```python
from build123d import *

# Parameters (mm, degrees)
SKETCH_1_W      = 20
SKETCH_1_H      = 20
EXTRUDE_1_DEPTH = 5
SKETCH_2_W      = 6
SKETCH_2_H      = 3
SKETCH_2_W_2    = 3
SKETCH_2_H_2    = 6
EXTRUDE_2_DEPTH = 15
SKETCH_3_W      = 6
SKETCH_3_H      = 3
EXTRUDE_3_DEPTH = 15
SKETCH_4_W      = 3
SKETCH_4_H      = 6
EXTRUDE_4_DEPTH = 15


with BuildPart() as part:
    # Эскиз1 → Бобышка-Вытянуть1 (new body)
    with BuildSketch(Plane.XY):
        with Locations((10, 10)):
            Rectangle(SKETCH_1_W, SKETCH_1_H)
    extrude(amount=EXTRUDE_1_DEPTH)

    # Эскиз2 → Бобышка-Вытянуть2 (add)
    with BuildSketch(Plane.XY.offset(5)):
        with Locations((10, 18.5)):
            Rectangle(SKETCH_2_W, SKETCH_2_H)
        with Locations((18.5, 10)):
            Rectangle(SKETCH_2_W_2, SKETCH_2_H_2)
    extrude(amount=EXTRUDE_2_DEPTH)

    # Эскиз3 → Бобышка-Вытянуть3 (add)
    with BuildSketch(Plane.XZ):
        with Locations((10, 1.5)):
            Rectangle(SKETCH_3_W, SKETCH_3_H)
    extrude(amount=EXTRUDE_3_DEPTH)

    # Эскиз4 → Бобышка-Вытянуть4 (add)
    with BuildSketch(Plane.ZY):
        with Locations((1.5, 10)):
            Rectangle(SKETCH_4_W, SKETCH_4_H)
    extrude(amount=EXTRUDE_4_DEPTH)


solid = part.part
```
The listing builds one solid part. Answer for the finished solid, in the listing's coordinates (mm). A direction names the side the tool comes from. Give positions to 0.01 mm unless a question says otherwise; leave off trailing zeros. Loops run counter-clockwise (first coordinate to the right, second up) from the corner with the lowest first, then second, coordinate; pieces in that order, holes last. Notation, with made-up numbers: (76, 26.25) - (108, 26.25) arc R22 ccw to (108, 37.25) - close; hole circle Ø7 at (71, 68.5). An arc over 180 degrees is marked (long way). Return JSON: item names as keys, results as strings. Group by question number.
1. Find section C-C (y = -6). Write down the section's boundary in (x, z).
2. Which of the six approach directions +Z, -Z, +X, -X, +Y, -Y give full straight-line access (tool end or side, diameter ignored) to faces 4 (the flat face through (18, 13, 12)), 5 (the flat face through (7, -7, 1)), 6 (the flat face through (7, 18, 12)), 7 (the flat face through (10, -7, 3))?
3. Given pin 1 Ø3 at (x, y) = (9.5, -5) entering from +Z; pin 2 Ø1.5 at (x, y) = (-3, 15.5) entering from -Z; pin 3 Ø0.9 at (x, z) = (18, 13.5) entering from +Y; pin 4 Ø1.5 at (x, z) = (18, 13) entering from -Y, each flat-ended and moving along its own axis, determine where each tip first touches the part or whether it passes through.
4. Find section B-B (x = 9). Write down the section's boundary in (y, z).
5. Straight lines are drawn through the part: line 1 (Y direction, x = 8.5, z = 15.25); line 2 (Z direction, x = 2, y = 18.5); line 3 (Y direction, x = 10, z = 4.5). For each, find the intervals that lie inside material, in ascending order. Write a range as [from, to].
6. Find section D-D (z = 3.5). Write down the section's boundary in (x, y), then the cut area to 3 significant figures.
7. Find section A-A (z = 6.25). Write down the section's boundary in (x, y), then the cut area to 3 significant figures.
8. Determine the mould class of faces 1 (the flat face through (10, 17, 12)), 2 (the flat face through (13, -7, 1)), 3 (the flat face through (-15, 10, 1)) for opening direction X: pulls with the +X half, pulls with the -X half, needs draft (parallel to the pull), parting line crosses it, or undercut.
Verdict:
{
 "1": {"outline": "(7, 0) - (13, 0) - (13, 3) - (7, 3) - close"},
 "2": {"face 4": "+Z, +X, -X, +Y", "face 5": "+Z, -Z, -X, -Y", "face 6": "+Z, -X, +Y, -Y", "face 7": "+Z, +X, -X, -Y"},
 "3": {"pin 1": "stops at z = 3", "pin 2": "passes through", "pin 3": "stops at y = 13", "pin 4": "stops at y = 7"},
 "4": {"outline": "(-15, 0) - (20, 0) - (20, 20) - (17, 20) - (17, 5) - (0, 5) - (0, 3) - (-15, 3) - close"},
 "5": {"line 1": "y = [17, 20]", "line 2": "z = [0, 5]", "line 3": "y = [0, 20]"},
 "6": {"outline": "(0, 0) - (20, 0) - (20, 20) - (0, 20) - close", "area": "400 mm^2"},
 "7": {"outline": "(7, 17) - (13, 17) - (13, 20) - (7, 20) - close; (17, 7) - (20, 7) - (20, 13) - (17, 13) - close", "area": "36.0 mm^2"},
 "8": {"face 1": "needs draft", "face 2": "pulls with the +X half", "face 3": "pulls with the -X half"}
}
